```python
from build123d import *

# Parameters (mm, degrees)
F1_DEPTH = 288
F2_R     = 2.54
F3_DEPTH = 50.8
F4_R     = 2.54
F5_DEPTH = 25.4


with BuildPart() as f1:
    # F0 (on Front) → F1 (new body)
    with BuildSketch(Plane.XZ):
        Polygon((-15, 15.75), (-16, 15.75), (-16, -16.25), (16, -16.25), (16, 15.75), (15, 15.75), (15, -15.25), (-15, -15.25), align=None)
    extrude(amount=F1_DEPTH)

    # F2 (on face) → F3 (cut)
    with BuildSketch(Plane(origin=(-16, 0, 0), x_dir=(0, -1, 0), z_dir=(-1, 0, 0))):
        with Locations((16, -0.25)):
            Circle(F2_R)
        with Locations((48, -0.25)):
            Circle(F2_R)
        with Locations((80, -0.25)):
            Circle(F2_R)
        with Locations((112, -0.25)):
            Circle(F2_R)
        with Locations((144, -0.25)):
            Circle(F2_R)
        with Locations((176, -0.25)):
            Circle(F2_R)
        with Locations((208, -0.25)):
            Circle(F2_R)
        with Locations((240, -0.25)):
            Circle(F2_R)
        with Locations((272, -0.25)):
            Circle(F2_R)
    extrude(amount=-F3_DEPTH, mode=Mode.SUBTRACT)

    # F4 (on face) → F5 (cut)
    with BuildSketch(Plane(origin=(0, 0, -16.25), x_dir=(1, 0, 0), z_dir=(0, 0, -1))):
        with Locations((0, 272)):
            Circle(F4_R)
        with Locations((0, 240)):
            Circle(F4_R)
        with Locations((0, 208)):
            Circle(F4_R)
        with Locations((0, 176)):
            Circle(F4_R)
        with Locations((0, 144)):
            Circle(F4_R)
        with Locations((0, 112)):
            Circle(F4_R)
        with Locations((0, 80)):
            Circle(F4_R)
        with Locations((0, 48)):
            Circle(F4_R)
        with Locations((0, 16)):
            Circle(F4_R)
    extrude(amount=-F5_DEPTH, mode=Mode.SUBTRACT)


solid = f1.part
```
Input: part model. Units: mm. Frame: model coordinates. Round coordinates to 2 decimals unless told otherwise and drop trailing zeros. Loops run counter-clockwise (first coordinate to the right, second up) from the corner with the lowest first, then second, coordinate; pieces in that order, holes last. Notation, with made-up numbers: M 45.25,-32.75 L 67.25,-32.75 A8 ccw 67.25,-18.75 Z; hole C 0,1.5 d11. An arc over 180 degrees is marked long. Answer in a Markdown table with one row per item. Add a question column.
1. Section B-B (z = -5.5). Output: boundary loops of the cut face in (x, y), and give its area (3 significant figures).
2. Section C-C (x = 0). Give the number of separate pieces and of enclosed holes in the cut face, and give its area (3 significant figures).
3. Mould query, pull axis X, two halves, no side actions, for faces 1 (the face through (-15.507, -45.462, -0.138)), 2 (the face through (1.37, -178.14, -15.76)). Classes: released by +X, released by -X, zero draft, split by the parting line, or undercut.
4. Section A-A (y = -80). Output: boundary loops of the cut face in (x, z), and give its area (3 significant figures).
5. Section D-D (y = -262). Output: boundary loops of the cut face in (x, z), and give its area (3 significant figures).
6. Ray query, probe 1 along X at (y, z) = (-23.5, 6.5); probe 2 along Z at (x, y) = (15.75, -272); probe 3 along Z at (x, y) = (13, -188.5). Return the intervals inside material, ascending.
7. Contact query for a flat-ended pin moving along its axis: pin 1 (9 mm diameter, centred on x = -1.5, y = -192, fed in from +Z). Output: stop coordinate, or through.
Values follow:
| question | item | result |
|---|---|---|
| 1 | outline | M -16,-288 L -15,-288 L -15,0 L -16,0 Z; M 15,-288 L 16,-288 L 16,0 L 15,0 Z |
| 1 | area | 576 mm^2 |
| 2 | separate pieces | 10 |
| 2 | enclosed holes | 0 |
| 2 | area | 242 mm^2 |
| 3 | face 1 | zero draft |
| 3 | face 2 | undercut |
| 4 | outline | M -16,-16.25 L -2.54,-16.25 L -2.54,-15.25 L -15,-15.25 L -15,-2.79 L -16,-2.79 Z; M -16,2.29 L -15,2.29 L -15,15.75 L -16,15.75 Z; M 2.54,-16.25 L 16,-16.25 L 16,-2.79 L 15,-2.79 L 15,-15.25 L 2.54,-15.25 Z; M 15,2.29 L 16,2.29 L 16,15.75 L 15,15.75 Z |
| 4 | area | 78.8 mm^2 |
| 5 | outline | M -16,-16.25 L 16,-16.25 L 16,15.75 L 15,15.75 L 15,-15.25 L -15,-15.25 L -15,15.75 L -16,15.75 Z |
| 5 | area | 94.0 mm^2 |
| 6 | probe 1 | -16 to -15, 15 to 16 |
| 6 | probe 2 | -16.25 to -2.79, 2.29 to 15.75 |
| 6 | probe 3 | -16.25 to -15.25 |
| 7 | pin 1 | z = -15.25 |
